from build123d import *

# Parameters (mm, degrees)
BOSS_EXTRUDE1_DEPTH = 3
FILLET1_R           = 20
SKETCH2_W           = 3
SKETCH2_H           = 7
SKETCH2_W_2         = 16
SKETCH2_H_2         = 3
SKETCH2_H_3         = 10
SKETCH2_H_4         = 12
CUT_EXTRUDE1_DEPTH  = 10
SKETCH3_R           = 10.816374358
SKETCH3_R_2         = 9.958860775
SKETCH3_R_3         = 9.948633444
SKETCH3_R_4         = 7.040136574
SKETCH3_R_5         = 5.125609119
SKETCH3_R_6         = 6.486312195
SKETCH3_R_7         = 5.814914906
SKETCH3_R_8         = 3.86625454
CUT_EXTRUDE2_DEPTH  = 10


with BuildPart() as part:
    # Sketch1 → Boss-Extrude1 (new body)
    with BuildSketch(Plane.XY):
        with BuildLine():
            Line((-0.5, -84.19), (0.5, -84.19))
            Line((0.5, -84.19), (25, -84.19))
            ThreePointArc((25, -84.19), (60.355339059, -69.545339059), (75, -34.19))
            Line((75, -34.19), (75, 63.81))
            ThreePointArc((75, 63.81), (71.192388155, 73.002388155), (62, 76.81))
            Line((62, 76.81), (-62, 76.81))
            ThreePointArc((-62, 76.81), (-71.192388155, 73.002388155), (-75, 63.81))
            Line((-75, 63.81), (-75, -34.19))
            ThreePointArc((-75, -34.19), (-60.355339059, -69.545339059), (-25, -84.19))
            Line((-25, -84.19), (-0.5, -84.19))
        make_face()
        with BuildLine():
            Line((50, 51.81), (-50, 51.81))
            Line((-50, 51.81), (-50, -34.19))
            ThreePointArc((-50, -34.19), (-42.67766953, -51.86766953), (-25, -59.19))
            Line((-25, -59.19), (-0.5, -59.19))
            Line((-0.5, -59.19), (0.5, -59.19))
            Line((0.5, -59.19), (25, -59.19))
            ThreePointArc((25, -59.19), (42.67766953, -51.86766953), (50, -34.19))
            Line((50, -34.19), (50, 51.81))
        make_face(mode=Mode.SUBTRACT)
    extrude(amount=BOSS_EXTRUDE1_DEPTH)

    # Fillet1
    fillet1_edges = [part.edges().sort_by_distance(p)[0] for p in [
        (50, 51.81, 1.5),
        (-50, 51.81, 1.5),
    ]]
    fillet(fillet1_edges, radius=FILLET1_R)

    # Sketch2 → Cut-Extrude1 (cut)
    with BuildSketch(Plane(origin=(0, 0, 0), x_dir=(-1, 0, 0), z_dir=(0, 0, -1))):
        with Locations((-10.5, 73.31)):
            Rectangle(SKETCH2_W, SKETCH2_H)
        with Locations((-10.5, -80.69)):
            Rectangle(SKETCH2_W, SKETCH2_H)
        with Locations((10.5, -80.69)):
            Rectangle(SKETCH2_W, SKETCH2_H)
        with Locations((10.5, 73.31)):
            Rectangle(SKETCH2_W, SKETCH2_H)
        with Locations((46, -62.69)):
            Rectangle(SKETCH2_W_2, SKETCH2_H_2)
        with Locations((-46, -62.69)):
            Rectangle(SKETCH2_W_2, SKETCH2_H_2)
        with Locations((28.5, -74.19)):
            Rectangle(SKETCH2_W, SKETCH2_H_3)
        with Locations((-28.5, -74.19)):
            Rectangle(SKETCH2_W, SKETCH2_H_3)
        with Locations((-73.5, 57.81)):
            Rectangle(SKETCH2_W, SKETCH2_H_4)
        with Locations((73.5, 57.81)):
            Rectangle(SKETCH2_W, SKETCH2_H_4)
    extrude(amount=-CUT_EXTRUDE1_DEPTH, mode=Mode.SUBTRACT)

    # Sketch3 → Cut-Extrude2 (cut)
    with BuildSketch(Plane(origin=(0, 0, 0), x_dir=(-1, 0, 0), z_dir=(0, 0, -1))):
        with Locations((-56.872719069, 60.521134432)):
            Circle(SKETCH3_R)
        with Locations((-62.296765207, 38.027296035)):
            Circle(SKETCH3_R_2)
        with Locations((-62.296765207, 13.459557643)):
            Circle(SKETCH3_R_2)
        with Locations(Location((-62.296765207, -38.027296035, 0), (0, 0, 180))):
            Circle(SKETCH3_R_2)
        with Locations(Location((-62.296765207, -13.459557643, 0), (0, 0, 180))):
            Circle(SKETCH3_R_2)
        with Locations((-32.2590485, 64.887956773)):
            Circle(SKETCH3_R_3)
        with Locations((-9.981507512, 61.202530051)):
            Circle(SKETCH3_R_4)
        with Locations((-61.336948944, -55.95327759)):
            Circle(SKETCH3_R_5)
        with Locations((-9.981507512, -67.886000723)):
            Circle(SKETCH3_R_6)
        with Locations((-40.143007857, -72.338509355)):
            Circle(SKETCH3_R_7)
        with Locations((-50.027577019, -53.727023274)):
            Circle(SKETCH3_R_8)
        with Locations(Location((50.027577019, -53.727023274, 0), (0, 0, 180))):
            Circle(SKETCH3_R_8)
        with Locations(Location((40.143007857, -72.338509355, 0), (0, 0, 180))):
            Circle(SKETCH3_R_7)
        with Locations(Location((9.981507512, -67.886000723, 0), (0, 0, 180))):
            Circle(SKETCH3_R_6)
        with Locations(Location((61.336948944, -55.95327759, 0), (0, 0, 180))):
            Circle(SKETCH3_R_5)
        with Locations(Location((9.981507512, 61.202530051, 0), (0, 0, 180))):
            Circle(SKETCH3_R_4)
        with Locations(Location((32.2590485, 64.887956773, 0), (0, 0, 180))):
            Circle(SKETCH3_R_3)
        with Locations((62.296765207, -13.459557643)):
            Circle(SKETCH3_R_2)
        with Locations((62.296765207, -38.027296035)):
            Circle(SKETCH3_R_2)
        with Locations(Location((62.296765207, 13.459557643, 0), (0, 0, 180))):
            Circle(SKETCH3_R_2)
        with Locations(Location((62.296765207, 38.027296035, 0), (0, 0, 180))):
            Circle(SKETCH3_R_2)
        with Locations(Location((56.872719069, 60.521134432, 0), (0, 0, 180))):
            Circle(SKETCH3_R)
    extrude(amount=-CUT_EXTRUDE2_DEPTH, mode=Mode.SUBTRACT)


solid = part.part
Part model, mm, in its own coordinate system. A direction names the side the tool comes from. Round coordinates to 2 decimals unless told otherwise and drop trailing zeros. Write each loop counter-clockwise with the first axis right and the second up, starting at its lowest first coordinate (ties: lowest second). Pieces come first, ordered by that corner, then holes. Notation, with made-up numbers: M 38.5,-9.75 L 67.5,-9.75 A20 ccw 67.5,7.25 Z; hole C 72,3 d3. An arc over 180 degrees is marked long. Return JSON: item names as keys, results as strings. Group by question number.
(1) Two-plate mould, pull along Y, no slides. Class faces 3 (the face through (52.8, 41.02, 1.48)), 4 (the face through (-60.7, -69.2, 1.5)), 5 (the face through (-50.4, -9.3, 3)): +Y half, -Y half, draft (parallel to the pull), parting line (faces both ways), or undercut.
(2) Which spindle directions (+Z, -Z, +X, -X, +Y, -Y) get a long thin tool onto all of the face, cutting with end or side? Do faces 1 (the face through (42.482, -52.061, 1.479)), 2 (the face through (71.293, 72.901, 1.479)). Say none if no direction does.
(3) Drill centre lines: probe 1 along Y at (x, z) = (19.5, 0.9); probe 2 along Y at (x, z) = (27.5, 2.9); probe 3 along Y at (x, z) = (47, 2.65). Where is each one in solid material? Low to high.
(4) Pin check, flat tips, straight feed: pin 1 Ø8 at (x, y) = (39.5, -67.5) entering from -Z; pin 2 Ø1.5 at (x, z) = (48, 1.5) entering from -Y; pin 3 Ø1.5 at (y, z) = (73.5, 1.5) entering from -X; pin 4 Ø0.9 at (x, z) = (29, 1.5) entering from -Y. Stop position of each tip, or through.
(5) Saw through at C-C on y = 18. Write the cut outline in (x, z).
(6) Saw through at A-A on y = -21. Write the cut outline in (x, z).
(7) Saw through at D-D on z = 1.2. Count the separate pieces of the cut face and the enclosed holes in it, then the cut area to 3 significant figures.
(8) Saw through at B-B on x = -40. Write the cut outline in (y, z).
Returned:
{
 "1": {"face 3": "undercut", "face 4": "-Y half", "face 5": "draft"},
 "2": {"face 1": "+Z, -Z", "face 2": "+Z, -Z, +X, +Y"},
 "3": {"probe 1": "-84.19 to -59.19, 51.81 to 76.81", "probe 2": "-84.13 to -79.19, -69.19 to -59.06, 51.81 to 56.15, 73.62 to 76.81", "probe 3": "-79.09 to -64.19, -61.19 to -56.13, -51.32 to -46.06, 42.35 to 56.1, 64.94 to 76.81"},
 "4": {"pin 1": "z = 0", "pin 2": "y = -78.97", "pin 3": "x = -71.44", "pin 4": "y = -84.06"},
 "5": {"outline": "M -75,0 L -71.16,0 L -71.16,3 L -75,3 Z; M -53.43,0 L -50,0 L -50,3 L -53.43,3 Z; M 50,0 L 53.43,0 L 53.43,3 L 50,3 Z; M 71.16,0 L 75,0 L 75,3 L 71.16,3 Z"},
 "6": {"outline": "M -75,0 L -68.8,0 L -68.8,3 L -75,3 Z; M -55.79,0 L -50,0 L -50,3 L -55.79,3 Z; M 50,0 L 55.79,0 L 55.79,3 L 50,3 Z; M 68.8,0 L 75,0 L 75,3 L 68.8,3 Z"},
 "7": {"separate pieces": "1", "enclosed holes": "27", "area": "7,140 mm²"},
 "8": {"outline": "M -81.89,0 L -78.15,0 L -78.15,3 L -81.89,3 Z; M -66.53,0 L -64.19,0 L -64.19,3 L -66.53,3 Z; M -61.19,0 L -54.19,0 L -54.19,3 L -61.19,3 Z; M 49.13,0 L 58.64,0 L 58.64,3 L 49.13,3 Z; M 71.14,0 L 76.81,0 L 76.81,3 L 71.14,3 Z"}
}
